Could you check a few things on this model? Use its own coordinates, in mm. Face numbers are marked on the shaded views. Give positions to 0.01 mm unless a question says otherwise; leave off trailing zeros. Write each loop counter-clockwise with the first axis right and the second up, starting at its lowest first coordinate (ties: lowest second). Pieces come first, ordered by that corner, then holes. Notation, with made-up numbers: (8.25, -9.5) -> (51.25, -9.5) arc R27 cw to (51.25, 20.5) -> close; hole circle Ø8 at (82, 35.25). An arc over 180 degrees is marked (long way). Write item = value, one per line. Start each with the question number.
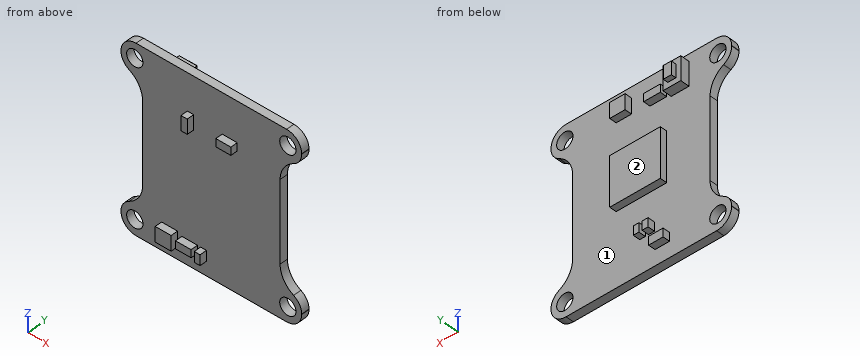
```python
from build123d import *

# Parameters (mm, degrees)
SKETCH1_R             = 1.625
PCB_DEPTH             = 1.6
SKETCH2_W             = 10.080807645
SKETCH2_H             = 9.766872459
SKETCH2_W_2           = 3.069588487
SKETCH2_H_2           = 3.0347068
SKETCH2_W_3           = 2.89518005
SKETCH2_H_3           = 1.674320993
SKETCH2_W_4           = 1.18597737
SKETCH2_H_4           = 1.744084367
SKETCH2_W_5           = 1.137538121
SKETCH2_H_5           = 1.77179178
SKETCH2_W_6           = 3.325937142
SKETCH2_H_6           = 1.560165557
TOP_COMPONENTS_DEPTH  = 1.4
FILLET1_R             = 3
FILLET2_R             = 5
SKETCH3_W             = 3.174233549
SKETCH3_H             = 2.964943425
SKETCH3_W_2           = 3.104470174
SKETCH3_H_2           = 1.534794244
SKETCH3_W_3           = 2.999825112
SKETCH3_H_3           = 1.569675931
SKETCH3_W_4           = 1.255740744
SKETCH3_H_4           = 2.895180051
SKETCH3_W_5           = 1.151095683
SKETCH3_H_5           = 2.058019554
REAR_COMPONENTS_DEPTH = 1.4
SKETCH4_W             = 3.55
SKETCH4_H             = 4.7
BUTTON_BASE_DEPTH     = 1.8
SKETCH5_W             = 1.6
SKETCH5_H             = 2.6
BUTTON_TIP_DEPTH      = 1


with BuildPart() as part:
    # Sketch1 → PCB (new body)
    with BuildSketch(Plane(origin=(0, 0, 0), x_dir=(1, 0, 0), z_dir=(0, 1, 0))):
        Polygon((-18, 18.2), (-18, 12.1), (-13.7, 12.1), (-13.7, -12.1), (-18, -12.1), (-18, -18.2), (18, -18.2), (18, -12.1), (13.7, -12.1), (13.7, 12.1), (18, 12.1), (18, 18.2), align=None)
        with Locations(Location((15.25, -15.25, 0), (0, 0, 270))):
            Circle(SKETCH1_R, mode=Mode.SUBTRACT)
        with Locations(Location((15.25, 15.25, 0), (0, 0, 270))):
            Circle(SKETCH1_R, mode=Mode.SUBTRACT)
        with Locations(Location((-15.25, 15.25, 0), (0, 0, 270))):
            Circle(SKETCH1_R, mode=Mode.SUBTRACT)
        with Locations(Location((-15.25, -15.25, 0), (0, 0, 270))):
            Circle(SKETCH1_R, mode=Mode.SUBTRACT)
    extrude(amount=PCB_DEPTH)

    # Sketch2 → Top components (add)
    with BuildSketch(Plane(origin=(0, 1.6, 0), x_dir=(1, 0, 0), z_dir=(0, 1, 0))):
        with Locations((-0.017440844, -1.151095683)):
            Rectangle(SKETCH2_W, SKETCH2_H)
        with Locations((3.488168735, -14.56310447)):
            Rectangle(SKETCH2_W_2, SKETCH2_H_2)
        with Locations((-4.168361639, 14.266610128)):
            Rectangle(SKETCH2_W_3, SKETCH2_H_3)
        with Locations((-2.023137867, 10.708678018)):
            Rectangle(SKETCH2_W_4, SKETCH2_H_4)
        with Locations((-0.233509749, 10.694824311)):
            Rectangle(SKETCH2_W_5, SKETCH2_H_5)
        with Locations((-3.394876095, -13.324858297)):
            Rectangle(SKETCH2_W_6, SKETCH2_H_6)
    extrude(amount=TOP_COMPONENTS_DEPTH)

    # Fillet1
    fillet1_edges = [part.edges().sort_by_distance(p)[0] for p in [
        (-18, 0.8, 18.2),
        (-18, 0.8, 12.1),
        (-18, 0.8, -12.1),
        (-18, 0.8, -18.2),
        (18, 0.8, -18.2),
        (18, 0.8, -12.1),
        (18, 0.8, 12.1),
        (18, 0.8, 18.2),
    ]]
    fillet(fillet1_edges, radius=FILLET1_R)

    # Fillet2
    fillet2_edges = [part.edges().sort_by_distance(p)[0] for p in [
        (13.7, 0.8, -12.1),
        (13.7, 0.8, 12.1),
        (-13.7, 0.8, 12.1),
        (-13.7, 0.8, -12.1),
    ]]
    fillet(fillet2_edges, radius=FILLET2_R)

    # Sketch3 → Rear components (add)
    with BuildSketch(Plane.XZ):
        with Locations((-8.319282433, -14.318932658)):
            Rectangle(SKETCH3_W, SKETCH3_H)
        with Locations((-4.307888388, -14.127083378)):
            Rectangle(SKETCH3_W_2, SKETCH3_H_2)
        with Locations((3.662577172, 9.540141492)):
            Rectangle(SKETCH3_W_3, SKETCH3_H_3)
        with Locations((-4.150920795, 9.470378117)):
            Rectangle(SKETCH3_W_4, SKETCH3_H_4)
        with Locations((-1.552235088, -14.388696033)):
            Rectangle(SKETCH3_W_5, SKETCH3_H_5)
    extrude(amount=REAR_COMPONENTS_DEPTH)

    # Sketch4 → Button base (add)
    with BuildSketch(Plane(origin=(0, 1.6, 0), x_dir=(1, 0, 0), z_dir=(0, 1, 0))):
        with Locations((-7.725, -14.45)):
            Rectangle(SKETCH4_W, SKETCH4_H)
    extrude(amount=BUTTON_BASE_DEPTH)

    # Sketch5 → Button tip (add)
    with BuildSketch(Plane(origin=(0, 3.4, 0), x_dir=(1, 0, 0), z_dir=(0, 1, 0))):
        with Locations((-7.725, -14.45)):
            Rectangle(SKETCH5_W, SKETCH5_H)
    extrude(amount=BUTTON_TIP_DEPTH)


solid = part.part
```
(1) I'm going to push flat-ended pins straight in: pin 1 (1.1 mm diameter, centred on x = 3, y = 2.5, fed in from -Z); pin 2 (5 mm diameter, centred on x = 15.25, z = 15.25, fed in from -Y); pin 3 (0.6 mm diameter, centred on x = -2, y = 2.5, fed in from +Z). Where does each tip first touch, or does it pass through?
(2) If I drill on line 1 along X through (y, z) = (0.7, 15.25) (3 decimals); line 2 along Z through (x, y) = (-2, 2.4); line 3 along Z through (x, y) = (-1.5, 1.65), over which ranges is the centre line in solid material (lowest first)? Write a range as from..to.
(3) Imagine slicing it at C-C (y = 0.75). State how many separate pieces and enclosed holes the cut face has, then the cut area to 3 significant figures.
(4) We'd pull the mould along Z, two halves only. Please class the marked faces 1 and 2: released by +Z, released by -Z, zero draft, split by the parting line, or undercut.
(5) Imagine slicing it at B-B (x = 10.5). Please give me the cut outline in (y, z).
(6) Imagine slicing it at A-A (z = -2). Please give me the cut outline in (x, y).
Answers below:
q1.pin_1 = -3.73
q1.pin_2 = 0
q1.pin_3 = 14.1
q2.line_1 = -18..-16.875, -13.625..13.625, 16.875..18
q2.line_2 = -11.58..-9.84, -3.73..6.03, 12.54..14.1
q2.line_3 = -11.58..-9.84, -3.73..6.03
q3.separate_pieces = 1
q3.enclosed_holes = 4
q3.area = 1,060 mm^2
q4.face_1 = undercut
q4.face_2 = zero draft
q5.outline = (0, -18.2) -> (1.6, -18.2) -> (1.6, 18.2) -> (0, 18.2) -> close
q6.outline = (-13.7, 0) -> (13.7, 0) -> (13.7, 1.6) -> (5.02, 1.6) -> (5.02, 3) -> (-5.06, 3) -> (-5.06, 1.6) -> (-13.7, 1.6) -> close
